Source: CAD feature listing. Evaluate the final solid. Frame: model axes, mm. A direction names the side the tool comes from. Give positions to 0.01 mm unless a question says otherwise; leave off trailing zeros. Order: outer loops, then holes, each group sorted by start corner. A loop starts at its lowest first (then second) coordinate and runs counter-clockwise, first axis right, second up. Notation, with made-up numbers: (-13, -33.75) - (33, -33.75) arc R16 ccw to (33, -13.75) - close; hole circle Ø6 at (-16, 59.5). An arc over 180 degrees is marked (long way). Use CSV: the item, a comma, the result in double quotes.
Autodesk Inventor part; units mm, degrees
ref_plane "YZ Plane" through (0, 0, 0) normal (1, 0, 0) x (0, 1, 0)
ref_plane "XZ Plane" through (0, 0, 0) normal (0, 1, 0) x (-1, 0, 0)
ref_plane "XY Plane" through (0, 0, 0) normal (0, 0, 1) x (1, 0, 0)
sketch "Эскиз1" plane through (0, 0, 0) normal (0, 0, 1) x (1, 0, 0)
  line L0 (0, 0) -> (30, 0)
  line L1 (30, 0) -> (30, 20)
  line L2 (30, 20) -> (0, 20)
  arc A0 (0.0661, 9) -> (0.0661, 11) centre (7.6, 10) ccw
  line L3 (0.0661, 11) -> (0, 11)
  line L4 (0.0661, 9) -> (0, 9)
  line L5 (0, 20) -> (0, 11)
  line L6 (0, 9) -> (0, 0)
  dimension "d0" = 30
  dimension "d1" = 20
extrude "Выдавливание1" add sketch "Эскиз1" along normal blind 58
sketch "Эскиз2" plane through (30, 0, 0) normal (1, 0, 0) x (0, 0, -1)
  circle A0 centre (-14.05, 10) radius 4.05
  line L0 (0, 20) -> (-58, 20)
  line L1 (-29, 20) -> (-29, 0)
  circle A1 centre (-43.95, 10) radius 4.05
  point P0 (0, 0)
  dimension "d4" = 8.1
extrude "Выдавливание2" cut sketch "Эскиз2" against normal blind 10
properties part number "x_holder"
Item 1: Section A-A on x = 7.6. Return the cut outline in (y, z), then the cut area to 3 significant figures.
Filled in:
outline,"(0, 0) - (2.4, 0) - (2.4, 58) - (0, 58) - close; (17.6, 0) - (20, 0) - (20, 58) - (17.6, 58) - close"
area,"278 mm2"
Item 2: First-contact query: pin 1 (6.5 mm diameter, centred on y = 10, z = 14.05, fed in from +X); pin 2 (1 mm diameter, centred on x = 6.5, y = 15.5, fed in from +Z). Flat tips, straight axial feed; report the tip coordinate or a pass-through.
Filled in:
pin 1,"stops at x = 20"
pin 2,"passes through"
Item 3: Section D-D on x = 24.75. Return the cut outline in (y, z).
Filled in:
outline,"(0, 0) - (20, 0) - (20, 58) - (0, 58) - close; hole circle Ø8.1 at (10, 14.05); hole circle Ø8.1 at (10, 43.95)"
Item 4: Set-up query: faces 1 (the flat face through (0, 16, 29)), 2 (the cylindrical face through (25.07, 8.45, 40.21)). Return all of +Z, -Z, +X, -X, +Y, -Y with unobstructed straight access to the full face (end or side cutting, diameter ignored); none if empty.
Filled in:
face 1,"+Z, -Z, -X, +Y, -Y"
face 2,"+X"
Item 5: Section C-C on y = 10. Return the cut outline in (x, z).
Filled in:
outline,"(15.2, 0) - (30, 0) - (30, 10) - (20, 10) - (20, 18.1) - (30, 18.1) - (30, 39.9) - (20, 39.9) - (20, 48) - (30, 48) - (30, 58) - (15.2, 58) - close"
Item 6: Material intervals for line 1 (Y direction, x = 27.25, z = 14.05); line 2 (Y direction, x = 7.6, z = 35); line 3 (Z direction, x = 27.25, y = 11.25), sorted ascending. Write a range as from..to.
Filled in:
line 1,"y = 0..5.95, 14.05..20"
line 2,"y = 0..2.4, 17.6..20"
line 3,"z = 0..10.2, 17.9..40.1, 47.8..58"
Item 7: Mould query, pull axis Z, two halves, no side actions, for faces 3 (the cylindrical face through (15.193, 10.32, 28.594)), 4 (the flat face through (18, 10, 58)), 5 (the flat face through (20, 10, 14)). Classes: released by +Z, released by -Z, zero draft, split by the parting line, or undercut.
Filled in:
face 3,"zero draft"
face 4,"released by +Z"
face 5,"undercut"
Item 8: Section B-B on z = 43.95. Return the cut outline in (x, y), then the cut area to 3 significant figures.
Filled in:
outline,"(0, 0) - (30, 0) - (30, 5.95) - (20, 5.95) - (20, 14.05) - (30, 14.05) - (30, 20) - (0, 20) - (0, 11) - (0.07, 11) arc R7.6 cw (long way) to (0.07, 9) - (0, 9) - close"
area,"337 mm2"
